Read the model definition and answer for the solid it produces. Units are mm, in the model's axes. A direction names the side the tool comes from. Give positions to 0.01 mm unless a question says otherwise; leave off trailing zeros. Order: outer loops, then holes, each group sorted by start corner. A loop starts at its lowest first (then second) coordinate and runs counter-clockwise, first axis right, second up. Notation, with made-up numbers: (-5, 87.5) -> (43, 87.5) arc R27 cw to (43, 126.5) -> close; hole circle Ø9 at (9.5, 72.5). An arc over 180 degrees is marked (long way). Use one line per item in the form item = value.
```python
from build123d import *

# Parameters (mm, degrees)
EXTRUDE_1_DEPTH     = 40
EXTRUDE_2_DEPTH     = 12
SKETCH_3_W          = 9.9
SKETCH_3_H          = 45.3
CUT_EXTRUDE_1_DEPTH = 10
SKETCH_4_W          = 3.5
SKETCH_4_H          = 35
CUT_EXTRUDE_2_DEPTH = 55.257079031
SKETCH_5_W          = 9.9
SKETCH_5_H          = 0.5
SKETCH_5_H_2        = 1
CUT_EXTRUDE_3_DEPTH = 6
SKETCH_6_R          = 1.15
CUT_EXTRUDE_4_DEPTH = 55.257079031
SKETCH_7_R          = 1.95
CUT_EXTRUDE_5_DEPTH = 1.2
SKETCH_10_R         = 1.15
CUT_EXTRUDE_6_DEPTH = 10
CUT_EXTRUDE_START   = -1
SKETCH_11_R         = 1.95
CUT_EXTRUDE_7_DEPTH = 10
SKETCH_12_W         = 5
SKETCH_12_H         = 3
CUT_EXTRUDE_8_DEPTH = 52.397671397


with BuildPart() as part:
    # 草图1 → 凸台-拉伸1 (new body)
    with BuildSketch(Plane(origin=(0, 0, 0), x_dir=(1, 0, 0), z_dir=(0, 1, 0))):
        Polygon((6.687916013, 5.137083987), (6, 13), (-6, 13), (-6.687916013, 5.137083987), (-11.825, 0), (11.825, 0), align=None)
    extrude(amount=EXTRUDE_1_DEPTH)

    # 草图2 → 凸台-拉伸2 (add)
    with BuildSketch(Plane(origin=(0, 40, 0), x_dir=(1, 0, 0), z_dir=(0, 1, 0))):
        Polygon((6.687916013, 5.137083987), (6, 13), (-6, 13), (-6.687916013, 5.137083987), (-6.687916013, 0), (6.687916013, 0), align=None)
    extrude(amount=EXTRUDE_2_DEPTH)

    # 草图3 → 切除-拉伸1 (cut)
    with BuildSketch(Plane.XY):
        with Locations((0, 27.35)):
            Rectangle(SKETCH_3_W, SKETCH_3_H)
    extrude(amount=-CUT_EXTRUDE_1_DEPTH, mode=Mode.SUBTRACT)

    # 草图4 → 切除-拉伸2 (cut, through all)
    with BuildSketch(Plane.XY.offset(-10)):
        with Locations((0, 27.35)):
            Rectangle(SKETCH_4_W, SKETCH_4_H)
    extrude(amount=-CUT_EXTRUDE_2_DEPTH, mode=Mode.SUBTRACT)

    # 草图5 → 切除-拉伸3 (cut)
    with BuildSketch(Plane.XY):
        with Locations((0, 50.25)):
            Rectangle(SKETCH_5_W, SKETCH_5_H)
        with Locations((0, 4.2)):
            Rectangle(SKETCH_5_W, SKETCH_5_H_2)
    extrude(amount=-CUT_EXTRUDE_3_DEPTH, mode=Mode.SUBTRACT)

    # 草图6 → 切除-拉伸4 (cut, through all)
    with BuildSketch(Plane.XY.offset(-10)):
        with Locations((0, 47.85)):
            Circle(SKETCH_6_R)
        with Locations(Location((0, 6.85, 0), (0, 0, 180))):
            Circle(SKETCH_6_R)
    extrude(amount=-CUT_EXTRUDE_4_DEPTH, mode=Mode.SUBTRACT)

    # 草图7 → 切除-拉伸5 (cut)
    with BuildSketch(Plane(origin=(0, 0, -13), x_dir=(-1, 0, 0), z_dir=(0, 0, -1))):
        with Locations((0, 47.85)):
            Circle(SKETCH_7_R)
        with Locations((0, 6.85)):
            Circle(SKETCH_7_R)
    extrude(amount=-CUT_EXTRUDE_5_DEPTH, mode=Mode.SUBTRACT)

    # 草图10 → 切除-拉伸6 (cut)
    with BuildSketch(Plane(origin=(-5.9125, 0, -5.9125), x_dir=(-0.7071067811865515, 0, 0.7071067811865437), z_dir=(-0.7071067811865437, 0, -0.7071067811865515))):
        with Locations((4.729070765, 36)):
            Circle(SKETCH_10_R)
        with Locations((4.729070765, 4)):
            Circle(SKETCH_10_R)
    cut_extrude_6 = extrude(amount=-CUT_EXTRUDE_6_DEPTH, mode=Mode.SUBTRACT)

    # 草图11 → 切除-拉伸7 (cut)
    with BuildSketch(Plane(origin=(-5.9125, 0, -5.9125), x_dir=(-0.7071067811865515, 0, 0.7071067811865437), z_dir=(-0.7071067811865437, 0, -0.7071067811865515)).offset(CUT_EXTRUDE_START)):
        with Locations((4.729070765, 36)):
            Circle(SKETCH_11_R)
        with Locations((4.729070765, 4)):
            Circle(SKETCH_11_R)
    cut_extrude_7 = extrude(amount=-CUT_EXTRUDE_7_DEPTH, mode=Mode.SUBTRACT)

    # 镜向1: 切除-拉伸6, 切除-拉伸7 across plane
    add(cut_extrude_6.mirror(Plane(origin=(0, 0, 0), x_dir=(0, 0, 1), z_dir=(1, 0, 0))), mode=Mode.SUBTRACT)
    add(cut_extrude_7.mirror(Plane(origin=(0, 0, 0), x_dir=(0, 0, 1), z_dir=(1, 0, 0))), mode=Mode.SUBTRACT)

    # 草图12 → 切除-拉伸8 (cut, through all)
    with BuildSketch(Plane(origin=(0, 3.7, 0), x_dir=(1, 0, 0), z_dir=(0, 1, 0))):
        with Locations((0, 1.5)):
            Rectangle(SKETCH_12_W, SKETCH_12_H)
    extrude(amount=-CUT_EXTRUDE_8_DEPTH, mode=Mode.SUBTRACT)


solid = part.part
```
Item 1: Given pin 1 Ø2.5 at (y, z) = (35.5, -11) entering from +X; pin 2 Ø2.5 at (y, z) = (25.5, -12) entering from -X; pin 3 Ø5 at (y, z) = (18, -11) entering from +X, each flat-ended and moving along its own axis, determine where each tip first touches the part or whether it passes through.
Checks:
pin_1 = 6.28
pin_2 = -6.2
pin_3 = 6.39
Item 2: The part is cut by section B-B on x = 0. State how many separate pieces and enclosed holes the cut face has, and give its area (3 significant figures).
Checks:
separate_pieces = 4
enclosed_holes = 0
area = 80.3 mm²
Item 3: Straight lines are drawn through the part: L1, parallel to Y at x = 0, z = -10.45; L2, parallel to Y at x = 0, z = -12.55; L3, parallel to Y at x = 1.25, z = -8. For each, find the intervals that lie inside material, in ascending order. Write a range as from..to.
Checks:
L1 = 0..5.7, 8..9.85, 44.85..46.7, 49..52
L2 = 0..4.9, 8.8..9.85, 44.85..45.9, 49.8..52
L3 = 0..4.7, 50..52
Item 4: The part is cut by section C-C on y = 20. Give the vertices of the cut face in (x, z) (3 decimals).
Checks:
outline = (-11.825, 0) -> (-6.688, -5.137) -> (-6, -13) -> (-1.75, -13) -> (-1.75, -10) -> (-4.95, -10) -> (-4.95, 0) -> close; (1.75, -13) -> (6, -13) -> (6.688, -5.137) -> (11.825, 0) -> (4.95, 0) -> (4.95, -10) -> (1.75, -10) -> close
Item 5: Determine the mould class of faces 1 (the flat face through (-8.84, 2.73, -1.57)), 2 (the cylindrical face through (0, 8, -11)), 3 (the flat face through (-1, 6, -11.8)) for opening direction Z: +Z half, -Z half, draft (parallel to the pull), parting line (faces both ways), or undercut.
Checks:
face_1 = undercut
face_2 = draft
face_3 = -Z half
Item 6: The part is cut by section D-D on x = 3.25. Give the vertices of the cut face in (y, z).
Checks:
outline = (0, -13) -> (52, -13) -> (52, 0) -> (50.5, 0) -> (50.5, -6) -> (50, -6) -> (50, -10) -> (4.7, -10) -> (4.7, -6) -> (3.7, -6) -> (3.7, 0) -> (0, 0) -> close
Item 7: The part is cut by section A-A on y = 47.85. Give the vertices of the cut face in (x, z).
Checks:
outline = (-6.69, -5.14) -> (-6, -13) -> (-1.95, -13) -> (-1.95, -11.8) -> (-1.15, -11.8) -> (-1.15, -10) -> (-4.95, -10) -> (-4.95, 0) -> (-6.69, 0) -> close; (1.15, -11.8) -> (1.95, -11.8) -> (1.95, -13) -> (6, -13) -> (6.69, -5.14) -> (6.69, 0) -> (4.95, 0) -> (4.95, -10) -> (1.15, -10) -> close
Item 8: Which of the six approach directions +Z, -Z, +X, -X, +Y, -Y give full straight-line access (tool end or side, diameter ignored) to faces 4 (the flat face through (-6.688, 46, -3)), 5 (the flat face through (-1.75, 27, -11)), 6 (the flat face through (8.84, 34.73, -1.57)), 7 (the flat face through (4.95, 27, -5))?
Checks:
face_4 = +Z, -Z, -X, +Y
face_5 = +Z, -Z
face_6 = none
face_7 = +Z
